Could you check a few things on this drawing? It's one solid part, dimensions in mm from its lowest x, y, z. A direction names the side the tool comes from. Round coordinates to 2 decimals unless told otherwise and drop trailing zeros. Write each loop counter-clockwise with the first axis right and the second up, starting at its lowest first coordinate (ties: lowest second). Pieces come first, ordered by that corner, then holes. Notation, with made-up numbers: (87, 0) -> (109, 0) arc R13 ccw to (109, 14) -> close; hole circle Ø5 at (25, 33). An arc over 180 degrees is marked (long way). Put each result on its own line as item: value. Start each with the question number.
1) If I drill on line 1 along X through (y, z) = (63.5, 7.5); line 2 along Z through (x, y) = (192, 98) (1 decimal); line 3 along Y through (x, z) = (44.5, 43.5), over which ranges is the centre line in solid material (lowest first)? Write a range as [from, to].
2) I want a section at D-D, the plane x = 120.5. List the corners of the cut face in (y, z) for me (1 decimal).
3) I want a section at A-A, the plane y = 40. List the corners of the cut face in (x, z) for me (1 decimal).
4) I want a section at B-B, the plane y = 107. List the corners of the cut face in (x, z) for me, then the cut area to 3 significant figures.
5) Will these pins go through, and if not, where does the flat tip stop? P1, Ø3, axis at x = 163.5, z = 56, coming from the +Y side; P2, Ø3, axis at y = 106, z = 11, coming from the +X side.
6) Which directions (+Z, -Z, +X, -X, +Y, -Y) give clear straight access to the entire face, cutting with the end or side of a thin tool? Please do the marked faces 1 and 2.
7) We'd pull the mould along Z, two halves only. Please class the marked faces 3, 4 and 5: released by +Z, released by -Z, zero draft, split by the parting line, or undercut.
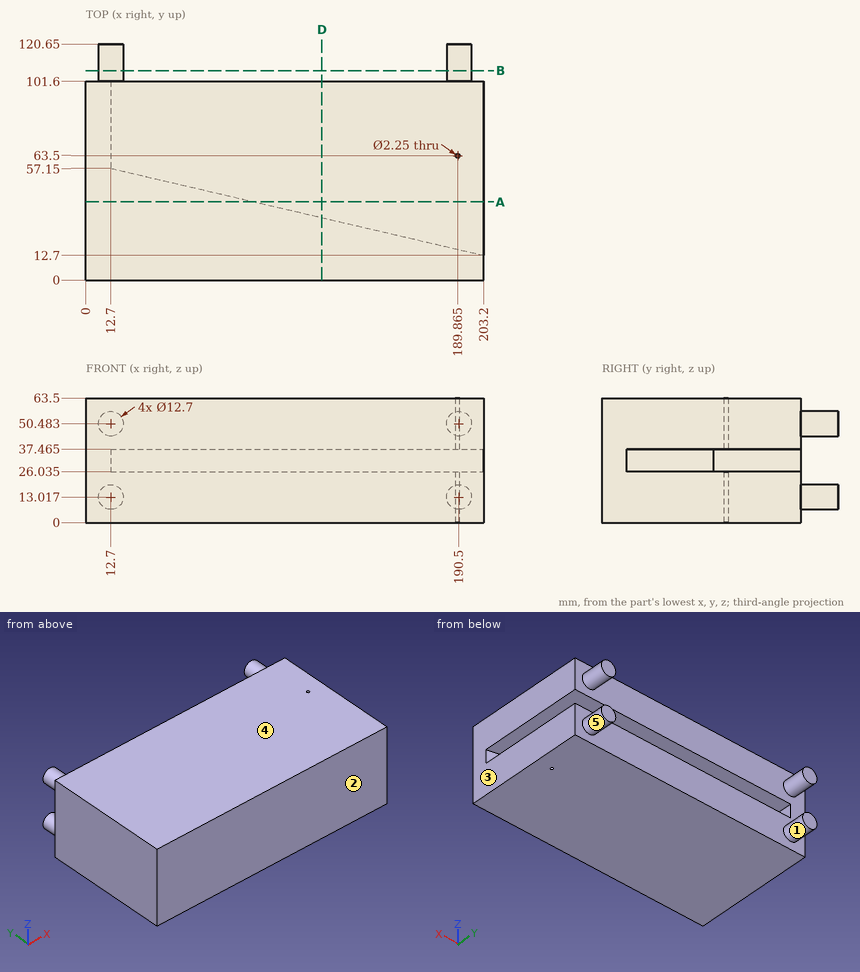
Findings:
1. line 1: x = [0, 188.74], [190.99, 203.2]
1. line 2: z = [0, 26], [37.5, 63.5]
1. line 3: y = [0, 101.6]
2. outline: (0, 0) -> (101.6, 0) -> (101.6, 26) -> (32, 26) -> (32, 37.5) -> (101.6, 37.5) -> (101.6, 63.5) -> (0, 63.5) -> close
3. outline: (0, 0) -> (203.2, 0) -> (203.2, 26) -> (86.2, 26) -> (86.2, 37.5) -> (203.2, 37.5) -> (203.2, 63.5) -> (0, 63.5) -> close
4. outline: circle Ø12.7 at (12.7, 13.02); circle Ø12.7 at (12.7, 50.48); circle Ø12.7 at (190.5, 13.02); circle Ø12.7 at (190.5, 50.48)
4. area: 507 mm2
5. P1: stops at y = 101.6
5. P2: stops at x = 196.83
6. face 1: +Y
6. face 2: +Z, -Z, +X, -X, -Y
7. face 3: zero draft
7. face 4: released by +Z
7. face 5: undercut
